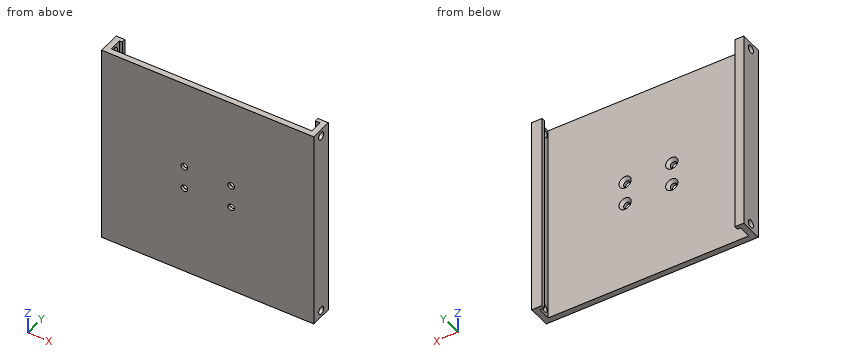
from build123d import *

# Parameters (mm, degrees)
BOSS_EXTRUDE1_DEPTH                            = 52.25
BOSS_EXTRUDE1_DEPTH_BACK                       = 52.25
CSK_FOR_M3_FLAT_HEAD_MACHINE_SCREW1_AT_2_COUNT = 2
CSK_FOR_M3_FLAT_HEAD_MACHINE_SCREW1_AT_2_PITCH = 12
CSK_FOR_M3_FLAT_HEAD_MACHINE_SCREW1_AT_3_COUNT = 2
CSK_FOR_M3_FLAT_HEAD_MACHINE_SCREW1_AT_3_PITCH = 26.83281573
CSK_FOR_M3_FLAT_HEAD_MACHINE_SCREW1_AT_4_COUNT = 2
CSK_FOR_M3_FLAT_HEAD_MACHINE_SCREW1_AT_4_PITCH = 24
SKETCH5_R                                      = 2
CUT_EXTRUDE1_DEPTH                             = 122.422042892


with BuildPart() as part:
    # Sketch1 → Boss-Extrude1 (new, two sides: drawn at the far end of the back side and taken through both)
    with BuildSketch(Plane.XY.offset(-BOSS_EXTRUDE1_DEPTH_BACK)):
        Polygon((-50, 11.5), (-50, 9.5), (-51.5, 9.5), (-51.5, 3), (51.5, 3), (51.5, 9.5), (49.2, 9.5), (49.2, 11.5), (54.5, 11.5), (54.5, 0), (-54.5, 0), (-54.5, 11.5), align=None)
    extrude(amount=BOSS_EXTRUDE1_DEPTH + BOSS_EXTRUDE1_DEPTH_BACK)

    # Sketch4 → CSK for M3 Flat Head Machine Screw1 (revolve, cut)
    with BuildSketch(Plane(origin=(-12, 3, -6), x_dir=(0, 0, 1), z_dir=(1, 0, 0))):
        Polygon((0, 0), (0, 3), (1.7, 3), (1.7, 1.45), (3.15, 0), align=None)
    csk_for_m3_flat_head_machine_screw1 = revolve(axis=Axis((-12, 9.35, -6), (0, -1, 0)), mode=Mode.SUBTRACT)

    # CSK for M3 Flat Head Machine Screw1 at 2: CSK for M3 Flat Head Machine Screw1 ×2
    with Locations(*[(0, 0, i * CSK_FOR_M3_FLAT_HEAD_MACHINE_SCREW1_AT_2_PITCH) for i in range(1, CSK_FOR_M3_FLAT_HEAD_MACHINE_SCREW1_AT_2_COUNT)]):
        add(csk_for_m3_flat_head_machine_screw1, mode=Mode.SUBTRACT)

    # CSK for M3 Flat Head Machine Screw1 at 3: CSK for M3 Flat Head Machine Screw1 ×2
    with Locations(*[Vector(0.894427190999916, 0, 0.4472135954999579) * (i * CSK_FOR_M3_FLAT_HEAD_MACHINE_SCREW1_AT_3_PITCH) for i in range(1, CSK_FOR_M3_FLAT_HEAD_MACHINE_SCREW1_AT_3_COUNT)]):
        add(csk_for_m3_flat_head_machine_screw1, mode=Mode.SUBTRACT)

    # CSK for M3 Flat Head Machine Screw1 at 4: CSK for M3 Flat Head Machine Screw1 ×2
    with Locations(*[(i * CSK_FOR_M3_FLAT_HEAD_MACHINE_SCREW1_AT_4_PITCH, 0, 0) for i in range(1, CSK_FOR_M3_FLAT_HEAD_MACHINE_SCREW1_AT_4_COUNT)]):
        add(csk_for_m3_flat_head_machine_screw1, mode=Mode.SUBTRACT)

    # Sketch5 → Cut-Extrude1 (cut, through all)
    with BuildSketch(Plane(origin=(54.5, 0, 0), x_dir=(0, 0, -1), z_dir=(1, 0, 0))):
        with Locations(Location((-48.75, 5.875, 0), (0, 0, 90))):
            Circle(SKETCH5_R)
        with Locations(Location((48.75, 5.875, 0), (0, 0, 90))):
            Circle(SKETCH5_R)
    extrude(amount=-CUT_EXTRUDE1_DEPTH, mode=Mode.SUBTRACT)


solid = part.part
The model under review builds one solid part; all positions refer to its coordinate system, in mm. Round coordinates to 2 decimals unless told otherwise and drop trailing zeros. Loops run counter-clockwise (first coordinate to the right, second up) from the corner with the lowest first, then second, coordinate; pieces in that order, holes last. Notation, with made-up numbers: (47, 0) -> (52, 0) arc R21 ccw to (52, 8) -> close; hole circle Ø3 at (-15, -11.75). An arc over 180 degrees is marked (long way). One line per question, with ' | ' between items. Start each with the question number.
Item 1: For pin 1 (2.5 mm diameter, centred on y = 5.875, z = 48.75, fed in from +X); pin 2 (4.5 mm diameter, centred on x = -12, z = 6, fed in from +Y), all flat-tipped, find the tip position at first contact; note any pin that passes through.
Item 2: Add section A-A, the plane z = 6. Write out the cut boundary in (x, y), then the cut area to 3 significant figures.
Item 3: Add section C-C, the plane y = 5.25. Write out the cut boundary in (x, z).
Item 4: Add section B-B, the plane x = 12. Write out the cut boundary in (y, z), then the cut area to 3 significant figures.
Item 5: Add section D-D, the plane z = -29. Write out the cut boundary in (x, y).
Item 6: Wall thickness on line 1 along X through (y, z) = (0.65, -6); line 2 along X through (y, z) = (10, 28); line 3 along X through (y, z) = (9, -16): over which ranges is each line inside the solid? List them lowest first. Write a range as [from, to].
Return value:
1) pin 1: passes through | pin 2: stops at y = 2.1
2) outline: (-54.5, 0) -> (-13.7, 0) -> (-13.7, 1.55) -> (-15.15, 3) -> (-51.5, 3) -> (-51.5, 9.5) -> (-50, 9.5) -> (-50, 11.5) -> (-54.5, 11.5) -> close; (-10.3, 0) -> (10.3, 0) -> (10.3, 1.55) -> (8.85, 3) -> (-8.85, 3) -> (-10.3, 1.55) -> close; (13.7, 0) -> (54.5, 0) -> (54.5, 11.5) -> (49.2, 11.5) -> (49.2, 9.5) -> (51.5, 9.5) -> (51.5, 3) -> (15.15, 3) -> (13.7, 1.55) -> close | area: 361 mm2
3) outline: (-54.5, -52.25) -> (-51.5, -52.25) -> (-51.5, -50.65) -> (-54.5, -50.65) -> close; (-54.5, -46.85) -> (-51.5, -46.85) -> (-51.5, 46.85) -> (-54.5, 46.85) -> close; (-54.5, 50.65) -> (-51.5, 50.65) -> (-51.5, 52.25) -> (-54.5, 52.25) -> close; (51.5, -52.25) -> (54.5, -52.25) -> (54.5, -50.65) -> (51.5, -50.65) -> close; (51.5, -46.85) -> (54.5, -46.85) -> (54.5, 46.85) -> (51.5, 46.85) -> close; (51.5, 50.65) -> (54.5, 50.65) -> (54.5, 52.25) -> (51.5, 52.25) -> close
4) outline: (0, -52.25) -> (3, -52.25) -> (3, -9.15) -> (1.55, -7.7) -> (0, -7.7) -> close; (0, -4.3) -> (1.55, -4.3) -> (3, -2.85) -> (3, 2.85) -> (1.55, 4.3) -> (0, 4.3) -> close; (0, 7.7) -> (1.55, 7.7) -> (3, 9.15) -> (3, 52.25) -> (0, 52.25) -> close | area: 289 mm2
5) outline: (-54.5, 0) -> (54.5, 0) -> (54.5, 11.5) -> (49.2, 11.5) -> (49.2, 9.5) -> (51.5, 9.5) -> (51.5, 3) -> (-51.5, 3) -> (-51.5, 9.5) -> (-50, 9.5) -> (-50, 11.5) -> (-54.5, 11.5) -> close
6) line 1: x = [-54.5, -13.7], [-10.3, 10.3], [13.7, 54.5] | line 2: x = [-54.5, -50], [49.2, 54.5] | line 3: x = [-54.5, -51.5], [51.5, 54.5]
